```python
from build123d import *

# Parameters (mm, degrees)
SKETCH_1_R          = 8.075
EXTRUDE_1_DEPTH     = 7
EXTRUDE_START       = -2
SKETCH_2_R          = 8.075
SKETCH_2_R_2        = 6.575
EXTRUDE_2_DEPTH     = 2
SKETCH_3_R          = 4
EXTRUDE_3_DEPTH     = 10
SKETCH_4_R          = 5
SKETCH_4_R_2        = 4
EXTRUDE_4_DEPTH     = 3
CHAMFER_1_SIZE      = 0.5
CUT_EXTRUDE_1_DEPTH = 7
CUT_EXTRUDE_2_DEPTH = 5
CUT_EXTRUDE_START   = -2
SKETCH_8_R          = 4
CUT_EXTRUDE_3_DEPTH = 2
FILLET_1_R          = 0.5
SKETCH_9_R          = 2.2
CUT_EXTRUDE_4_DEPTH = 10
EXTRUDE_START_2     = 3
SKETCH_10_R         = 10.075
SKETCH_10_R_2       = 8.075
EXTRUDE_5_DEPTH     = 3


with BuildPart() as part:
    # 草图1 → 凸台-拉伸1 (new body)
    with BuildSketch(Plane.XY):
        with BuildLine():
            ThreePointArc((0.395882675, 11.067922204), (-11.074999998, -0.000217919), (0.396318234, -11.067906616))
            Line((0.396318234, -11.067906616), (114, -7))
            ThreePointArc((114, -7), (120.998881523, -0.125129643), (114.250219298, 6.995526449))
            Line((114.250219298, 6.995526449), (0.395882675, 11.067922204))
        make_face()
        Circle(SKETCH_1_R, mode=Mode.SUBTRACT)
    extrude(amount=EXTRUDE_1_DEPTH)

    # 草图2 → 凸台-拉伸2 (add)
    with BuildSketch(Plane.XY.offset(7).offset(EXTRUDE_START)):
        Circle(SKETCH_2_R)
        Circle(SKETCH_2_R_2, mode=Mode.SUBTRACT)
    extrude(amount=EXTRUDE_2_DEPTH)

    # 草图3 → 凸台-拉伸3 (add)
    with BuildSketch(Plane(origin=(0, 0, 0), x_dir=(-1, 0, 0), z_dir=(0, 0, -1))):
        with Locations((-114, 0)):
            Circle(SKETCH_3_R)
    extrude(amount=EXTRUDE_3_DEPTH)

    # 草图4 → 凸台-拉伸4 (add)
    with BuildSketch(Plane(origin=(0, 0, 0), x_dir=(-1, 0, 0), z_dir=(0, 0, -1))):
        with Locations(Location((-114, 0, 0), (0, 0, 180))):
            Circle(SKETCH_4_R)
        with Locations((-114, 0)):
            Circle(SKETCH_4_R_2, mode=Mode.SUBTRACT)
    extrude(amount=EXTRUDE_4_DEPTH)

    # 倒角1
    chamfer_1_edges = [part.edges().sort_by_distance(p)[0] for p in [
        (-6.575, 0, 5),
        (-6.575, 0, 7),
        (118, 0, -10),
        (109, 0, -3),
    ]]
    chamfer(chamfer_1_edges, length=CHAMFER_1_SIZE)

    # 草图5 → 切除-拉伸1 (cut)
    with BuildSketch(Plane(origin=(0, 0, 0), x_dir=(-1, 0, 0), z_dir=(0, 0, -1))):
        with BuildLine():
            ThreePointArc((-12.757234161, -4.640431182), (-13.574999998, 0.000234775), (-12.757073645, 4.640872443))
            Line((-12.757073645, 4.640872443), (-104.114755838, 1.510611753))
            ThreePointArc((-104.114755838, 1.510611753), (-104.028730231, 0.75748214), (-104, 0))
            ThreePointArc((-104, 0), (-104.028593207, -0.755676237), (-104.114209315, -1.507031033))
            Line((-104.114209315, -1.507031033), (-12.757234161, -4.640431182))
        make_face()
    extrude(amount=-CUT_EXTRUDE_1_DEPTH, mode=Mode.SUBTRACT)

    # 草图6 → 切除-拉伸2 (cut)
    with BuildSketch(Plane(origin=(0, 0, 0), x_dir=(-1, 0, 0), z_dir=(0, 0, -1))):
        Polygon((-104.114209315, -1.507031033), (-12.757234161, -4.640431182), (-12.860068961, -7.638668165), (-104.217044114, -4.505268015), align=None)
        Polygon((-12.757073645, 4.640872443), (-104.114755838, 1.510611753), (-104.217486931, 4.508852291), (-12.859804737, 7.63911298), align=None)
    extrude(amount=-CUT_EXTRUDE_2_DEPTH, mode=Mode.SUBTRACT)

    # 草图8 → 切除-拉伸3 (cut)
    with BuildSketch(Plane(origin=(0, 0, -10), x_dir=(-1, 0, 0), z_dir=(0, 0, -1)).offset(CUT_EXTRUDE_START)):
        with Locations((-114, 0)):
            Circle(SKETCH_8_R)
    extrude(amount=CUT_EXTRUDE_3_DEPTH, mode=Mode.SUBTRACT)

    # 圆角1
    fillet_1_edges = [part.edges().sort_by_distance(p)[0] for p in [
        (118, 0, -8),
    ]]
    fillet(fillet_1_edges, radius=FILLET_1_R)

    # 草图9 → 切除-拉伸4 (cut)
    with BuildSketch(Plane(origin=(0, 0, -8), x_dir=(-1, 0, 0), z_dir=(0, 0, -1))):
        with Locations((-114, 0)):
            Circle(SKETCH_9_R)
    extrude(amount=-CUT_EXTRUDE_4_DEPTH, mode=Mode.SUBTRACT)

    # 草图10 → 凸台-拉伸5 (add)
    with BuildSketch(Plane(origin=(0, 0, 0), x_dir=(-1, 0, 0), z_dir=(0, 0, -1)).offset(EXTRUDE_START_2)):
        with Locations(Location((0, 0, 0), (0, 0, 180))):
            Circle(SKETCH_10_R)
        Circle(SKETCH_10_R_2, mode=Mode.SUBTRACT)
    extrude(amount=-EXTRUDE_5_DEPTH)

    # 切除-旋转2: read off the stored shape, not the designer's step
    # 切除-旋转2: loft between two sections, ruled curve by curve
    cut_revolve_2_from = [
        Edge.make_three_point_arc((8.65, 0, -1.2), (0, 8.65, -1.2), (-8.65, 0, -1.2)),
        Edge.make_three_point_arc((-8.65, 0, -1.2), (0, -8.65, -1.2), (8.65, 0, -1.2)),
    ]
    cut_revolve_2_to = [
        Edge.make_three_point_arc((8.65, 0, 0), (0, 8.65, 0), (-8.65, 0, 0)),
        Edge.make_three_point_arc((-8.65, 0, 0), (0, -8.65, 0), (8.65, 0, 0)),
    ]
    cut_revolve_2 = Solid(Shell([*[Face.make_surface_from_curves(cut_revolve_2_from[k], cut_revolve_2_to[k]) for k in range(2)], Face(Wire(cut_revolve_2_from)), Face(Wire(cut_revolve_2_to))]))
    add(cut_revolve_2, mode=Mode.SUBTRACT)


solid = part.part
```
Can you work these out from the model? Positions are in its coordinate system, mm. A direction names the side the tool comes from. Give positions to 0.01 mm unless a question says otherwise; leave off trailing zeros. Loops run counter-clockwise (first coordinate to the right, second up) from the corner with the lowest first, then second, coordinate; pieces in that order, holes last. Notation, with made-up numbers: M 89,41.5 L 94,41.5 A15 cw 94,63.5 Z; hole C 76.25,7 d8. An arc over 180 degrees is marked long. One line per question, with ' | ' between items. Start each with the question number.
Q1. If we mould it in two halves opening along X, with no side actions, what happens to faces 4 (the flat face through (58, 5, 5)), 5 (the flat face through (54, -5, 7)), 6 (the cylindrical face through (110.305, -1.532, -5.219))? For each: +X half, -X half, draft (parallel to the pull), parting line (faces both ways), or undercut.
Q2. For faces 1 (the flat face through (6, -6, -1.2)), 2 (the flat face through (-8, -3, -3)), 3 (the cylindrical face through (-7.995, 6.13, -1.521)), which set-ups out of +Z, -Z, +X, -X, +Y, -Y let a thin tool reach every point of the face, with its end or its side?
Q3. If we section it at B-B (x = 100): Please give me the cut outline in (y, z).
Q4. For pin 1 Ø1.3 at (x, y) = (113, 0.5) entering from -Z; pin 2 Ø13 at (x, y) = (0, 0) entering from +Z; pin 3 Ø1 at (y, z) = (7, -3) entering from +X; pin 4 Ø2 at (y, z) = (6.5, -3.5) entering from +X, each with a flat end and sliding along its axis, tell me the tip position at first contact or that it passes through.
Q5. If I drill on line 1 (Z direction, x = 8, y = -3); line 2 (X direction, y = 4, z = 2.5); line 3 (Z direction, x = 65.5, y = 3.5), over which ranges is the centre line in solid material (lowest first)? Write a range as from..to.
Q6. If we section it at A-A (x = 51.5): Please give me the cut outline in (y, z).
Computed:
1) face 4: undercut | face 5: draft | face 6: parting line
2) face 1: none | face 2: -Z, -X, +Y, -Y | face 3: -Z
3) outline: M -7.5,0 L -4.65,0 L -4.65,5 L -1.65,5 L -1.65,7 L -7.5,7 Z; M 1.65,5 L 4.65,5 L 4.65,0 L 7.51,0 L 7.51,7 L 1.65,7 Z
4) pin 1: stops at z = 2 | pin 2: passes through | pin 3: stops at x = 7.7 | pin 4: stops at x = 8.35
5) line 1: z = -3..-1.2, 0..7 | line 2: x = -10.33..-7.01, 7.01..12.97, 104.2..119.74 | line 3: z = 5..7
6) outline: M -9.24,0 L -6.31,0 L -6.31,5 L -3.31,5 L -3.31,7 L -9.24,7 Z; M 3.31,5 L 6.32,5 L 6.32,0 L 9.24,0 L 9.24,7 L 3.31,7 Z
